Work out the finished part from the listing and answer in its coordinate system (mm). Coordinates: 2 decimals unless noted, no trailing zeros. Loops run counter-clockwise (first coordinate to the right, second up) from the corner with the lowest first, then second, coordinate; pieces in that order, holes last. Notation, with made-up numbers: (70, -7) -> (104, -7) arc R19 cw to (104, 30) -> close; hole circle Ø1 at (29.5, 2.5). An arc over 180 degrees is marked (long way). Use a Markdown table: item, result.
Autodesk Inventor part; units mm, degrees
ref_plane "YZ Plane" through (0, 0, 0) normal (1, 0, 0) x (0, 1, 0)
ref_plane "XZ Plane" through (0, 0, 0) normal (0, 1, 0) x (-1, 0, 0)
ref_plane "XY Plane" through (0, 0, 0) normal (0, 0, 1) x (1, 0, 0)
sketch "Sketch1" plane through (0, 0, 0) normal (0, 1, 0) x (-1, 0, 0)
  line L0 (-75, 25) -> (75, 25)
  line L1 (75, 25) -> (75, -25)
  line L2 (75, -25) -> (-75, -25)
  line L3 (-75, -25) -> (-75, 25)
  line L4 (-75, 25) -> (75, -25) construction
  line L5 (75, 25) -> (-75, -25) construction
  line L6 (-75, -25) -> (-35, -25)
  line L7 (-35, -25) -> (-35, 25)
  line L8 (-35, 25) -> (-75, 25)
  line L9 (-75, 25) -> (-75, -25)
  line L10 (-35, 25) -> (-35, 75)
  line L11 (-35, 75) -> (75, 75)
  line L12 (75, 75) -> (75, 25)
  line L13 (-35, 75) -> (25, 75)
  line L14 (25, 75) -> (75, 25)
  point P0 (0, 0)
  point P1 (-35, -25)
  dimension "d0" = 150
  dimension "d1" = 50
  dimension "d57" = 40
  dimension "d58" = 50
  dimension "d59" = 50
  dimension "d60" = 60
extrude "Extrusion1" add sketch "Sketch1" along normal blind 3 contours L10 L11 L14 L0 | L0 L1 L2 L7
sketch "Sketch6" plane through (0, 3, 0) normal (0, 1, 0) x (1, 0, 0)
  line L0 (35, 25) -> (-75, 25)
  line L1 (0, 25) -> (0, 8)
  circle A0 centre (0, 8) radius 5.25
  line L2 (0, 8) -> (-53.4, 8)
  circle A1 centre (-53.4, 8) radius 5
  circle A2 centre (0, 8) radius 8
  circle A3 centre (0, 16) radius 1.75
  circle A4 centre (-8, 8) radius 1.75
  circle A5 centre (0, 0) radius 1.75
  circle A6 centre (8, 8) radius 1.75
  circle A7 centre (-53.4, 8) radius 12
  line L3 (-53.4, -4) -> (-53.4, 20)
  circle A8 centre (-53.4, 20) radius 1.75
  circle A9 centre (-65.4, 8) radius 1.75
  circle A10 centre (-53.4, -4) radius 1.75
  circle A11 centre (-41.4, 8) radius 1.75
  point P0 (0, 0)
  point P1 (75, 25)
  dimension "d49" = 24
  dimension "d40" = 17
  dimension "d41" = 10.5
  dimension "d42" = 53.4
  dimension "d43" = 10
  dimension "d44" = 3.5
  dimension "d47" = 360
  dimension "d50" = 3.5
  dimension "d53" = 360
extrude "Extrusion6" cut sketch "Sketch6" against normal through all contours A3 A2 L1 | A11 A7 L2 | L2 A7 A11 | L1 A2 A3 | A2 A3 L1 | L1 A3 A2 | A4 L2 A2 | A2 L2 A4 | A0 L2 L1 | L1 L2 A0 | A6 A2 | A2 A6 | A2 A4 L2 | L2 A4 A2 | A5 A2 | A2 A5 | A7 A11 L2 | L2 A11 A7 | A8 L3 A7 | A7 A8 | A10 A7 | A7 L3 A10 | A1 L3 L2 | L2 L3 A1 | L3 A8 A7 | A7 A10 L3 | L3 A1 | A9 A7 | A7 A9
fillet "Fillet1" radius 20 5 edges at (35, 1.5, -25) (35, 1.5, 75) (-25, 1.5, 75) (-75, 1.5, 25) (-75, 1.5, -25)
sketch "Sketch7" plane through (0, 3, 0) normal (0, 1, 0) x (1, 0, 0)
  arc A0 (15, -75) -> (35, -55) centre (15, -55) ccw
  line L0 (35, -55) -> (0, -55)
  line L1 (-16.7157, -75) -> (15, -75)
  line L2 (0, -75) -> (0, -35.4)
  line L3 (0, -75) -> (39.6, -75) construction
  circle A1 centre (0, -35.4) radius 26.5
  circle A2 centre (0, -61.9) radius 2.15
  circle A3 centre (26.5, -35.4) radius 2.15
  circle A4 centre (0, -8.9) radius 2.15
  circle A5 centre (-26.5, -35.4) radius 2.15
  point P0 (0, 0)
  dimension "d65" = 53
  dimension "d62" = 35
  dimension "d63" = 39.6
  dimension "d64" = 90
  dimension "d66" = 4.3
  dimension "d69" = 360
extrude "Extrusion7" cut sketch "Sketch7" against normal through all contours A2 A1 L2 | L2 A1 A2 | A1 L2 A2 | A3 A1 | A1 A3 | A1 A2 L2 | A5 A1 | A1 A5 | A4 A1 | A1 A4
properties part number "TopMount"
Q1. Given pin 1 Ø1 at (y, z) = (1.5, -13.5) entering from -X, flat-ended and moving along its own axis, determine where the tip first touches the part or whether it passes through.
Solved:
| item | result |
|---|---|
| pin 1 | x = -73.33 |
Q2. Section B-B on x = -8 is taken. Determine the outline of the cut face in (y, z), and give its area (4 significant figures).
Solved:
| item | result |
|---|---|
| outline | (0, -25) -> (3, -25) -> (3, -9.75) -> (0, -9.75) -> close; (0, -6.25) -> (3, -6.25) -> (3, 75) -> (0, 75) -> close |
| area | 289.5 mm² |
Q3. Consider line 1 (Z direction, x = 0, y = 2.1); line 2 (X direction, y = 1.8, z = 4); line 3 (X direction, y = 0.3, z = -5). Determine where each line is inside the solid, lowest interval first. Write a range as [from, to].
Solved:
| item | result |
|---|---|
| line 1 | [-25, -17.75], [-14.25, -13.25], [-2.75, -1.75], [1.75, 6.75], [11.05, 59.75], [64.05, 75] |
| line 2 | [-75, -55.15], [-51.65, 35] |
| line 3 | [-75, -57.4], [-49.4, -4.31], [4.31, 35] |
Q4. Determine the mould class of faces 1 (the cylindrical face through (-24.471, 1.521, 73.435)), 2 (the flat face through (35, 1, 25)), 3 (the flat face through (-19, 3, 26)), 4 (the cylindrical face through (-53.628, 1.521, -21.735)) for opening direction X: pulls with the +X half, pulls with the -X half, needs draft (parallel to the pull), parting line crosses it, or undercut.
Solved:
| item | result |
|---|---|
| face 1 | pulls with the -X half |
| face 2 | pulls with the +X half |
| face 3 | needs draft |
| face 4 | undercut |
Q5. Section D-D on y = 1.85 is taken. State how many separate pieces and enclosed holes the cut face has, and give its area (3 significant figures).
Solved:
| item | result |
|---|---|
| separate pieces | 1 |
| enclosed holes | 14 |
| area | 9,180 mm² |
Q6. Section A-A on z = 4 is taken. Determine the outline of the cut face in (x, y), and give its area (4 significant figures).
Solved:
| item | result |
|---|---|
| outline | (-75, 0) -> (-55.15, 0) -> (-55.15, 3) -> (-75, 3) -> close; (-51.65, 0) -> (35, 0) -> (35, 3) -> (-51.65, 3) -> close |
| area | 319.5 mm² |
Q7. Section C-C on x = -53.4 is taken. Determine the outline of the cut face in (y, z), and give its area (3 significant figures).
Solved:
| item | result |
|---|---|
| outline | (0, -25) -> (3, -25) -> (3, -21.75) -> (0, -21.75) -> close; (0, -18.25) -> (3, -18.25) -> (3, -13) -> (0, -13) -> close; (0, -3) -> (3, -3) -> (3, 2.25) -> (0, 2.25) -> close; (0, 5.75) -> (3, 5.75) -> (3, 46.6) -> (0, 46.6) -> close |
| area | 164 mm² |
